Build history of the part. All positions in model axes, mm. A direction names the side the tool comes from. Give positions to 0.01 mm unless a question says otherwise; leave off trailing zeros. Loops run counter-clockwise (first coordinate to the right, second up) from the corner with the lowest first, then second, coordinate; pieces in that order, holes last. Notation, with made-up numbers: (-13.75, 72.5) -> (12.25, 72.5) arc R23 cw to (12.25, 85.5) -> close; hole circle Ø3 at (41.25, -30). An arc over 180 degrees is marked (long way). Answer as a JSON object with one key per item and string values. Group by question number.
Q1. Band-saw the part on C-C, the plane y = 12. Write the cut outline in (x, z) (3 decimals).
Q2. Band-saw the part on B-B, the plane z = -31.75. Write the cut outline in (x, y) (3 decimals), plus the area to 3 significant figures.
Q3. Band-saw the part on D-D, the plane z = -2.5. Write the cut outline in (x, y) (3 decimals), plus the area to 3 significant figures.
Q4. Wall check: probe 1 along X at (y, z) = (5.5, -31.75) (3 decimals); probe 2 along X at (y, z) = (24.25, -29.5); probe 3 along Z at (x, y) = (55, 9.25). Give the ranges that are in metal, low to high. Write a range as from..to.
Q5. Band-saw the part on A-A, the plane x = 45. Write the cut outline in (y, z) (3 decimals), plus the area to 3 significant figures.
Q6. Two-plate mould, pull along X, no slides. Class faces 1 (the flat face through (0, 14, -22)), 2 (the flat face through (81.28, 14, -22)), 3 (the flat face through (40, 14, -44.45)), 4 (the flat face through (4.811, 15.114, -4.714)): pulls with the +X half, pulls with the -X half, needs draft (parallel to the pull), parting line crosses it, or undercut.
Q7. Drop flat-ended pins along their axis: pin 1 (8 mm diameter, centred on y = 16.5, z = -23.5, fed in from -X); pin 2 (2.5 mm diameter, centred on x = 78.28, z = -3, fed in from +Y); pin 3 (1.5 mm diameter, centred on x = 21, z = -39, fed in from +Y); pin 4 (4.5 mm diameter, centred on x = 66.5, z = -29.5, fed in from +Y). Give the stop position or say it passes through.
Q8. Tool access for faces 5 (the flat face through (40, 14, 0)), 6 (the cylindrical face through (72.89, 5.78, -17.18)): list every direction of +Z, -Z, +X, -X, +Y, -Y with a clear straight run to the whole face (end or side of a thin tool).
from build123d import *

# Parameters (mm, degrees)
SKETCH1_W           = 81.28
SKETCH1_H           = 44.45
BOSS_EXTRUDE1_DEPTH = 28.575
SHELL1_T            = -1.27
CHAMFER1_SIZE       = 6.985
SKETCH2_R           = 1.5
CUT_EXTRUDE1_DEPTH  = 97.947261565
SKETCH3_R           = 3.175
SKETCH3_R_2         = 4.445
SKETCH3_W           = 4
SKETCH3_H           = 12
SKETCH3_W_2         = 16.764
SKETCH3_H_2         = 12.192
CUT_EXTRUDE2_DEPTH  = 97.580556661
BOSS_EXTRUDE2_START = 8.89
SKETCH4_R           = 5.715
SKETCH4_R_2         = 4.445
SKETCH4_R_3         = 3.175
BOSS_EXTRUDE2_DEPTH = 8.89


with BuildPart() as part:
    # Sketch1 → Boss-Extrude1 (new body)
    with BuildSketch(Plane(origin=(0, 0, 0), x_dir=(1, 0, 0), z_dir=(0, 1, 0))):
        with Locations((40.64, 22.225)):
            Rectangle(SKETCH1_W, SKETCH1_H)
    extrude(amount=BOSS_EXTRUDE1_DEPTH)

    # Shell1
    shell1_openings = [part.faces().sort_by_distance(p)[0] for p in [
        (40.64, 28.575, -22.225),
    ]]
    offset(amount=SHELL1_T, openings=shell1_openings, kind=Kind.INTERSECTION)

    # Chamfer1
    chamfer1_edges = [part.edges().sort_by_distance(p)[0] for p in [
        (1.27, 14.9225, -43.18),
        (1.27, 14.9225, -1.27),
        (80.01, 14.9225, -1.27),
        (80.01, 14.9225, -43.18),
    ]]
    chamfer(chamfer1_edges, length=CHAMFER1_SIZE)

    # Sketch2 → Cut-Extrude1 (cut, through all)
    with BuildSketch(Plane(origin=(0, 28.575, 0), x_dir=(1, 0, 0), z_dir=(0, 1, 0))):
        with Locations(Location((3, 41.45, 0), (0, 0, 270))):
            Circle(SKETCH2_R)
        with Locations(Location((3, 3, 0), (0, 0, 270))):
            Circle(SKETCH2_R)
        with Locations(Location((78.28, 3, 0), (0, 0, 270))):
            Circle(SKETCH2_R)
        with Locations(Location((78.28, 41.45, 0), (0, 0, 270))):
            Circle(SKETCH2_R)
    extrude(amount=-CUT_EXTRUDE1_DEPTH, mode=Mode.SUBTRACT)

    # Sketch3 → Cut-Extrude2 (cut, through all)
    with BuildSketch(Plane(origin=(0, 1.27, 0), x_dir=(1, 0, 0), z_dir=(0, 1, 0))):
        with Locations(Location((67.31, 31.75, 0), (0, 0, 270))):
            Circle(SKETCH3_R)
        with Locations(Location((67.31, 18.415, 0), (0, 0, 270))):
            Circle(SKETCH3_R_2)
        with Locations((7.62, 22.225)):
            Rectangle(SKETCH3_W, SKETCH3_H)
        with Locations((40.64, 22.225)):
            Rectangle(SKETCH3_W_2, SKETCH3_H_2)
    extrude(amount=-CUT_EXTRUDE2_DEPTH, mode=Mode.SUBTRACT)

    # Sketch4 → Boss-Extrude2 (add)
    # profile 1 of 2: a face of its own
    with BuildSketch(Plane(origin=(0, 1.27, 0), x_dir=(1, 0, 0), z_dir=(0, 1, 0)).offset(BOSS_EXTRUDE2_START)):
        with Locations(Location((67.31, 18.415, 0), (0, 0, 90))):
            Circle(SKETCH4_R)
        with Locations(Location((67.31, 18.415, 0), (0, 0, 270))):
            Circle(SKETCH4_R_2, mode=Mode.SUBTRACT)
    # profile 2 of 2: a face of its own
    with BuildSketch(Plane(origin=(0, 1.27, 0), x_dir=(1, 0, 0), z_dir=(0, 1, 0)).offset(BOSS_EXTRUDE2_START)):
        with Locations(Location((67.31, 31.75, 0), (0, 0, 90))):
            Circle(SKETCH4_R_2)
        with Locations(Location((67.31, 31.75, 0), (0, 0, 270))):
            Circle(SKETCH4_R_3, mode=Mode.SUBTRACT)
    extrude(amount=-BOSS_EXTRUDE2_DEPTH)


solid = part.part
Worked answers:
{
 "1": {"outline": "(0, -44.45) -> (81.28, -44.45) -> (81.28, 0) -> (0, 0) -> close; hole (1.27, -36.195) -> (8.255, -43.18) -> (73.025, -43.18) -> (80.01, -36.195) -> (80.01, -8.255) -> (73.025, -1.27) -> (8.255, -1.27) -> (1.27, -8.255) -> close; hole circle Ø3 at (3, -41.45); hole circle Ø3 at (3, -3); hole circle Ø3 at (78.28, -41.45); hole circle Ø3 at (78.28, -3)"},
 "2": {"outline": "(0, 0) -> (64.135, 0) -> (64.135, 10.16) -> (62.865, 10.16) -> (62.865, 1.27) -> (1.27, 1.27) -> (1.27, 28.575) -> (0, 28.575) -> close; (70.485, 0) -> (81.28, 0) -> (81.28, 28.575) -> (80.01, 28.575) -> (80.01, 1.27) -> (71.755, 1.27) -> (71.755, 10.16) -> (70.485, 10.16) -> close", "area": "187 mm2"},
 "3": {"outline": "(0, 0) -> (1.586, 0) -> (1.586, 28.575) -> (0, 28.575) -> close; (4.414, 0) -> (76.866, 0) -> (76.866, 28.575) -> (74.255, 28.575) -> (74.255, 1.27) -> (7.025, 1.27) -> (7.025, 28.575) -> (4.414, 28.575) -> close; (79.694, 0) -> (81.28, 0) -> (81.28, 28.575) -> (79.694, 28.575) -> close", "area": "325 mm2"},
 "4": {"probe 1": "0..1.27, 62.865..64.135, 70.485..71.755, 80.01..81.28", "probe 2": "0..1.27, 80.01..81.28", "probe 3": "-44.45..-43.18, -1.27..0"},
 "5": {"outline": "(0, -44.45) -> (28.575, -44.45) -> (28.575, -43.18) -> (1.27, -43.18) -> (1.27, -28.321) -> (0, -28.321) -> close; (0, -16.129) -> (1.27, -16.129) -> (1.27, -1.27) -> (28.575, -1.27) -> (28.575, 0) -> (0, 0) -> close", "area": "110 mm2"},
 "6": {"face 1": "pulls with the -X half", "face 2": "pulls with the +X half", "face 3": "needs draft", "face 4": "undercut"},
 "7": {"pin 1": "x = 0", "pin 2": "through", "pin 3": "y = 1.27", "pin 4": "y = 10.16"},
 "8": {"face 5": "+Z, +X, -X, +Y, -Y", "face 6": "+Y"}
}
